```python
from build123d import *

# Parameters (mm, degrees)
SKETCH1_W            = 161
SKETCH1_H            = 46
SKETCH1_R            = 1.825
SKETCH1_R_2          = 3.5
BOSS_EXTRUDE1_DEPTH  = 4
SKETCH2_W            = 49.5
SKETCH2_H            = 46
SKETCH2_W_2          = 30
SKETCH2_H_2          = 15
SKETCH2_W_3          = 44.5
BOSS_EXTRUDE2_DEPTH  = 4
M5_CLEARANCE_HOLE1_D = 5.5


with BuildPart() as part:
    # Sketch1 → Boss-Extrude1 (new body)
    with BuildSketch(Plane.XY):
        Rectangle(SKETCH1_W, SKETCH1_H)
        with Locations((-75.5, 13)):
            Circle(SKETCH1_R, mode=Mode.SUBTRACT)
        with Locations((-44.5, 13)):
            Circle(SKETCH1_R, mode=Mode.SUBTRACT)
        with Locations((-75.5, -18)):
            Circle(SKETCH1_R, mode=Mode.SUBTRACT)
        with Locations((-44.5, -18)):
            Circle(SKETCH1_R, mode=Mode.SUBTRACT)
        with Locations((60, -2.5)):
            Circle(SKETCH1_R_2, mode=Mode.SUBTRACT)
        with Locations((-15.5, 13)):
            Circle(SKETCH1_R, mode=Mode.SUBTRACT)
        with Locations((15.5, 13)):
            Circle(SKETCH1_R, mode=Mode.SUBTRACT)
        with Locations((-15.5, -18)):
            Circle(SKETCH1_R, mode=Mode.SUBTRACT)
        with Locations((15.5, -18)):
            Circle(SKETCH1_R, mode=Mode.SUBTRACT)
        with Locations((44.5, -18)):
            Circle(SKETCH1_R, mode=Mode.SUBTRACT)
        with Locations((75.5, -18)):
            Circle(SKETCH1_R, mode=Mode.SUBTRACT)
        with Locations((-60, -2.5)):
            Circle(SKETCH1_R_2, mode=Mode.SUBTRACT)
        with Locations((0, -2.5)):
            Circle(SKETCH1_R_2, mode=Mode.SUBTRACT)
        with Locations((44.5, 13)):
            Circle(SKETCH1_R, mode=Mode.SUBTRACT)
        with Locations((75.5, 13)):
            Circle(SKETCH1_R, mode=Mode.SUBTRACT)
    extrude(amount=BOSS_EXTRUDE1_DEPTH)

    # Sketch2 → Boss-Extrude2 (add)
    with BuildSketch(Plane.XY.offset(4)):
        with Locations((-105.25, 0)):
            Rectangle(SKETCH2_W, SKETCH2_H)
        with Locations((-115, -30.5)):
            Rectangle(SKETCH2_W_2, SKETCH2_H_2)
        with Locations((102.75, 0)):
            Rectangle(SKETCH2_W_3, SKETCH2_H)
        with Locations((110, -30.5)):
            Rectangle(SKETCH2_W_2, SKETCH2_H_2)
    extrude(amount=-BOSS_EXTRUDE2_DEPTH)

    # M5 Clearance Hole1 (through all)
    with Locations(Plane.XY.offset(4)):
        with Locations((-115, -1.5), (-115, -26.5), (110, -1.5), (110, -26.5), (-115, 11), (110, 11), (110, -14), (-115, -14)):
            Hole(M5_CLEARANCE_HOLE1_D / 2)


solid = part.part
```
For this review, take the finished solid that the model builds, in its own axes (mm). A direction names the side the tool comes from. Coordinates: 2 decimals unless noted, no trailing zeros. Write each loop counter-clockwise with the first axis right and the second up, starting at its lowest first coordinate (ties: lowest second). Pieces come first, ordered by that corner, then holes.
(1) Wall thickness on probe 1 along X at (y, z) = (-14.5, 2.25); probe 2 along Y at (x, z) = (-75.5, 2.5) (3 decimals); probe 3 along Y at (x, z) = (-115, 3.1): over which ranges is each line inside the solid? List them lowest first.
(2) Add section D-D on y = -14. Give the boundary of the cut face in (x, z), then the cut area to 3 significant figures.
(3) The part is to be moulded in two halves that separate along Y. For faces 1 (the face through (125, -8, 2)), 2 (the face through (-0.759, -5.917, 1.972)), 3 (the face through (110, -38, 2)), say which applies: +Y half, -Y half, draft (parallel to the pull), parting line (faces both ways), or undercut.
(4) Add section C-C on x = -60. Give the boundary of the cut face in (y, z), then the cut area to 3 significant figures.
(5) Tool access review of faces 4 (the face through (112.747, -13.879, 1.972)), 5 (the face through (-100, -31, 2)): name each direction out of +Z, -Z, +X, -X, +Y, -Y from which nothing blocks a thin tool from reaching the whole face with its end or side.
(6) Add section B-B on z = 2. Count the separate pieces of the cut face and the enclosed holes in it, then the cut area to 3 significant figures.
(7) For pin 1 Ø5.5 at (x, y) = (0, -2.5) entering from -Z; pin 2 Ø2 at (x, z) = (-65, 2.5) entering from -Y, all flat-tipped, find the tip position at first contact; note any pin that passes through.
(8) Add section A-A on y = -26.5. Give the boundary of the cut face in (x, z), then the cut area to 3 significant figures.
Answer sheet:
1. probe 1: x = -130 to -117.7, -112.3 to 107.3, 112.7 to 125
1. probe 2: y = -23 to -19.825, -16.175 to 11.175, 14.825 to 23
1. probe 3: y = -38 to -29.25, -23.75 to -16.75, -11.25 to -4.25, 1.25 to 8.25, 13.75 to 23
2. outline: (-130, 0) - (-117.75, 0) - (-117.75, 4) - (-130, 4) - close; (-112.25, 0) - (107.25, 0) - (107.25, 4) - (-112.25, 4) - close; (112.75, 0) - (125, 0) - (125, 4) - (112.75, 4) - close
2. area: 976 mm2
3. face 1: draft
3. face 2: undercut
3. face 3: -Y half
4. outline: (-23, 0) - (-6, 0) - (-6, 4) - (-23, 4) - close; (1, 0) - (23, 0) - (23, 4) - (1, 4) - close
4. area: 156 mm2
5. face 4: +Z, -Z
5. face 5: +Z, -Z, -Y
6. separate pieces: 1
6. enclosed holes: 23
6. area: 12,200 mm2
7. pin 1: passes through
7. pin 2: stops at y = -23
8. outline: (-130, 0) - (-117.75, 0) - (-117.75, 4) - (-130, 4) - close; (-112.25, 0) - (-100, 0) - (-100, 4) - (-112.25, 4) - close; (95, 0) - (107.25, 0) - (107.25, 4) - (95, 4) - close; (112.75, 0) - (125, 0) - (125, 4) - (112.75, 4) - close
8. area: 196 mm2
